The drawing under review shows one solid part. Ordinate dimensions are in mm from its lowest x, y, z. A direction names the side the tool comes from. Give positions to 0.01 mm unless a question says otherwise; leave off trailing zeros. Order: outer loops, then holes, each group sorted by start corner. A loop starts at its lowest first (then second) coordinate and runs counter-clockwise, first axis right, second up. Notation, with made-up numbers: M -26,-30.5 L -15,-30.5 A17 cw -15,-20.5 Z; hole C -26.75,-24 d2. An arc over 180 degrees is marked long. Put each result on its own line as item: value. Start each with the question number.
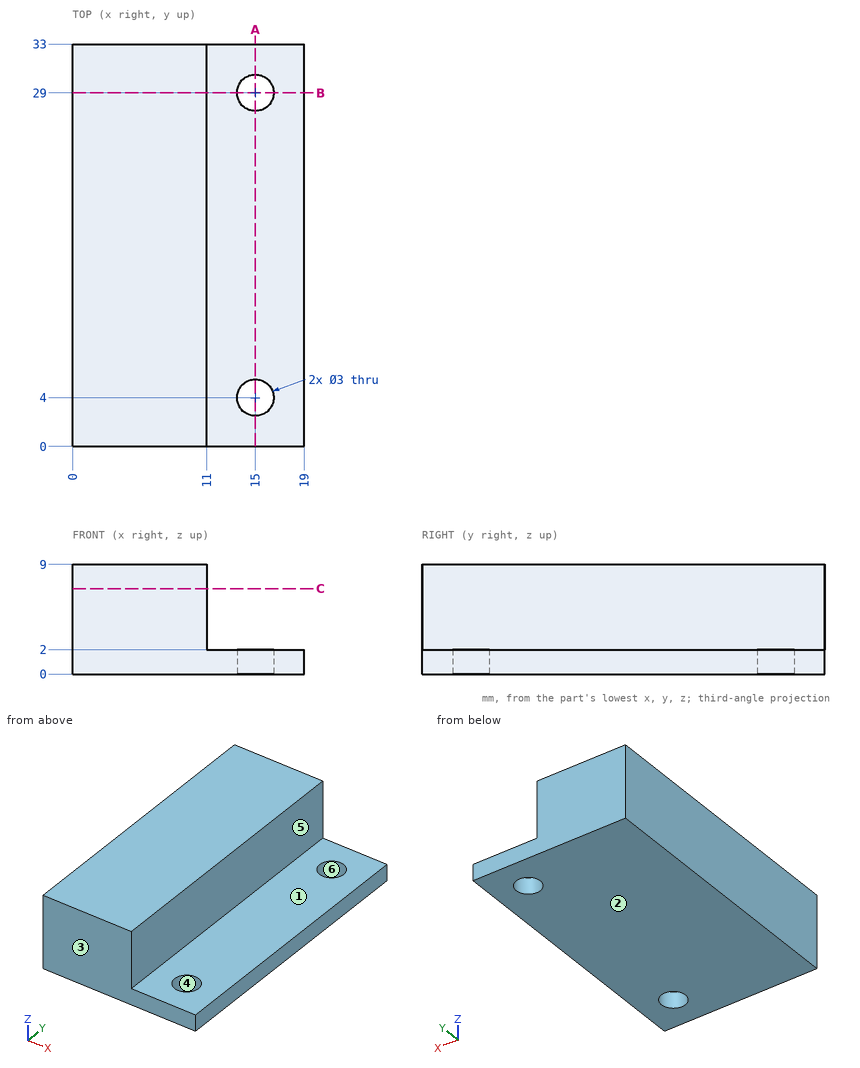
1. The part is to be moulded in two halves that separate along X. For the marked faces 3, 4, 5 and 6, say which applies: +X half, -X half, draft (parallel to the pull), parting line (faces both ways), or undercut.
2. Insertion check: pin 1 (9 mm diameter, centred on x = 13.5, y = 11.5, fed in from +Z); pin 2 (2.5 mm diameter, centred on x = 15, y = 4, fed in from +Z); pin 3 (4 mm diameter, centred on x = 16.5, y = 20.5, fed in from +Z). Each pin has a flat end and moves straight along its axis. Give the tip position at first contact, or say it passes through.
3. Consider section A-A on x = 15. Give the boundary of the cut face in (y, z), then the cut area to 3 significant figures.
4. Machinability: for the marked faces 1 and 2, which of the approach directions +Z, -Z, +X, -X, +Y, -Y give a long, thin tool a straight path to every point of the face, cutting with its end or side? Answer none if there is none.
5. Consider section B-B on y = 29. Give the boundary of the cut face in (x, z), then the cut area to 3 significant figures.
6. Consider section C-C on z = 7. Give the boundary of the cut face in (x, y).
7. To check wall thickness, follow probe 1 along Y at (x, z) = (15, 1); probe 2 along Z at (x, y) = (13.5, 29.5); probe 3 along X at (y, z) = (30, 1.25). State the ranges of each line that lie inside material, in increasing order.
Returned:
1. face 3: draft
1. face 4: undercut
1. face 5: +X half
1. face 6: undercut
2. pin 1: stops at z = 9
2. pin 2: passes through
2. pin 3: stops at z = 2
3. outline: M 0,0 L 2.5,0 L 2.5,2 L 0,2 Z; M 5.5,0 L 27.5,0 L 27.5,2 L 5.5,2 Z; M 30.5,0 L 33,0 L 33,2 L 30.5,2 Z
3. area: 54.0 mm2
4. face 1: +Z, +X, +Y, -Y
4. face 2: -Z, +X, -X, +Y, -Y
5. outline: M 0,0 L 13.5,0 L 13.5,2 L 11,2 L 11,9 L 0,9 Z; M 16.5,0 L 19,0 L 19,2 L 16.5,2 Z
5. area: 109 mm2
6. outline: M 0,0 L 11,0 L 11,33 L 0,33 Z
7. probe 1: y = 0 to 2.5, 5.5 to 27.5, 30.5 to 33
7. probe 2: z = 0 to 2
7. probe 3: x = 0 to 13.88, 16.12 to 19
